Work out the finished part from the listing and answer in its coordinate system (mm). A direction names the side the tool comes from. Give positions to 0.01 mm unless a question says otherwise; leave off trailing zeros. Order: outer loops, then holes, each group sorted by start corner. A loop starts at its lowest first (then second) coordinate and runs counter-clockwise, first axis right, second up. Notation, with made-up numbers: (50.25, 20) -> (102.25, 20) arc R29 ccw to (102.25, 53) -> close; hole circle Ø3 at (-39.5, -26.5). An arc over 180 degrees is marked (long way). Use a Markdown table: item, result. Add a question column.
```python
from build123d import *

# Parameters (mm, degrees)
SKETCH1_W           = 135
SKETCH1_H           = 122
BOSS_EXTRUDE1_DEPTH = 5.7
CUT_EXTRUDE1_DEPTH  = 57


with BuildPart() as part:
    # Sketch1 → Boss-Extrude1 (new body)
    with BuildSketch(Plane(origin=(0, 0, 0), x_dir=(0, 0, -1), z_dir=(1, 0, 0))):
        with Locations((67.5, 61)):
            Rectangle(SKETCH1_W, SKETCH1_H)
    extrude(amount=BOSS_EXTRUDE1_DEPTH)

    # Sketch2 → Cut-Extrude1 (cut)
    with BuildSketch(Plane(origin=(0, 0, 0), x_dir=(0, 0, -1), z_dir=(1, 0, 0))):
        Polygon((0, 116), (27, 116), (27, 121.7), (54, 121.7), (54, 116), (81, 116), (81, 121.7), (108, 121.7), (108, 116), (135, 116), (135, 130), (0, 130), align=None)
        Polygon((0, -8), (0, 6), (27, 6), (27, 0.3), (54, 0.3), (54, 6), (81, 6), (81, 0.3), (108, 0.3), (108, 6), (135, 6), (135, -8), align=None)
    extrude(amount=CUT_EXTRUDE1_DEPTH, mode=Mode.SUBTRACT)


solid = part.part
```
1) Which of the six approach directions +Z, -Z, +X, -X, +Y, -Y give full straight-line access (tool end or side, diameter ignored) to faces 4 (the flat face through (3, 116, -13)), 5 (the flat face through (3, 119, -108)), 6 (the flat face through (3, 6, -121)), 7 (the flat face through (3, 119, -81))?
2) Straight lines are drawn through the part: line 1 (Y direction, x = 1.4, z = -119.5); line 2 (Z direction, x = 1.4, y = 116.5). For each, find the intervals that lie inside material, in ascending order.
3) Flat-ended cylindrical pins translate along their axes: pin 1 (3 mm diameter, centred on x = 2.5, y = 2.5, fed in from -Z); pin 2 (1.7 mm diameter, centred on x = 1.5, y = 117.5, fed in from +Z); pin 3 (3 mm diameter, centred on x = 2.5, z = -120.5, fed in from +Y). Find the tip coordinate at first contact, or state that the pin passes through.
4) Determine the mould class of faces 1 (the flat face through (3, 3, -27)), 2 (the flat face through (3, 119, -54)), 3 (the flat face through (3, 0.3, -40)) for opening direction Z: released by +Z, released by -Z, zero draft, split by the parting line, or undercut.
5) The part is cut by section A-A, the plane x = 3.85. Determine the outline of the cut face in (y, z).
6) The part is cut by section B-B, the plane z = -124.5. Determine the outline of the cut face in (x, y).
A:
| question | item | result |
|---|---|---|
| 1 | face 4 | +Z, +X, -X, +Y |
| 1 | face 5 | -Z, +X, -X, +Y |
| 1 | face 6 | -Z, +X, -X, -Y |
| 1 | face 7 | +X, -X, +Y |
| 2 | line 1 | 6 to 116 |
| 2 | line 2 | -108 to -81, -54 to -27 |
| 3 | pin 1 | z = -108 |
| 3 | pin 2 | z = -27 |
| 3 | pin 3 | y = 116 |
| 4 | face 1 | released by +Z |
| 4 | face 2 | undercut |
| 4 | face 3 | zero draft |
| 5 | outline | (0.3, -108) -> (6, -108) -> (6, -135) -> (116, -135) -> (116, -108) -> (121.7, -108) -> (121.7, -81) -> (116, -81) -> (116, -54) -> (121.7, -54) -> (121.7, -27) -> (116, -27) -> (116, 0) -> (6, 0) -> (6, -27) -> (0.3, -27) -> (0.3, -54) -> (6, -54) -> (6, -81) -> (0.3, -81) -> close |
| 6 | outline | (0, 6) -> (5.7, 6) -> (5.7, 116) -> (0, 116) -> close |
